```python
from build123d import *

# Parameters (mm, degrees)
SKETCH2_R           = 136
BOSS_EXTRUDE1_DEPTH = 8
SKETCH3_R           = 111.5
SKETCH3_R_2         = 108.5
CUT_EXTRUDE1_DEPTH  = 2
SKETCH4_R           = 3.3
CUT_EXTRUDE2_DEPTH  = 22
CIRPATTERN1_COUNT   = 6
SKETCH6_R           = 67.5
SKETCH6_R_2         = 55
BOSS_EXTRUDE2_DEPTH = 10
SKETCH7_R           = 3.3
CUT_EXTRUDE3_DEPTH  = 15
CIRPATTERN2_COUNT   = 6


with BuildPart() as part:
    # Sketch1 → Revolve1 (revolve)
    with BuildSketch(Plane.XY, mode=Mode.PRIVATE) as revolve1_sk:
        with BuildLine():
            Line((-65, 0), (-65, 5))
            Line((-65, 5), (-54.772255751, 5))
            ThreePointArc((-54.772255751, 5), (-37.080992435, 40.620192023), (0, 55))
            Line((0, 55), (0, 50))
            ThreePointArc((0, 50), (-35.355339059, 35.355339059), (-50, 0))
            Line((-50, 0), (-65, 0))
        make_face()
    revolve(revolve1_sk.sketch.rotate(Axis((0, 0, 0), (0, 1, 0)), 180), axis=Axis((0, 0, 0), (0, 1, 0)))

    # Sketch2 → Boss-Extrude1 (add)
    with BuildSketch(Plane(origin=(0, 0, 0), x_dir=(1, 0, 0), z_dir=(0, 1, 0))):
        with Locations(Location((0, 0, 0), (0, 0, 270))):
            Circle(SKETCH2_R)
    extrude(amount=BOSS_EXTRUDE1_DEPTH)

    # Sketch3 → Cut-Extrude1 (cut)
    with BuildSketch(Plane(origin=(0, 0, 0), x_dir=(1, 0, 0), z_dir=(0, 1, 0))):
        with Locations(Location((0, 0, 0), (0, 0, 180))):
            Circle(SKETCH3_R)
        with Locations(Location((0, 0, 0), (0, 0, 180))):
            Circle(SKETCH3_R_2, mode=Mode.SUBTRACT)
    extrude(amount=CUT_EXTRUDE1_DEPTH, mode=Mode.SUBTRACT)

    # Sketch4 → Cut-Extrude2 (cut)
    with BuildSketch(Plane(origin=(0, 0, 0), x_dir=(-1, 0, 0), z_dir=(0, -1, 0))):
        with Locations(Location((0, 121, 0), (0, 0, 180))):
            Circle(SKETCH4_R)
    cut_extrude2 = extrude(amount=-CUT_EXTRUDE2_DEPTH, mode=Mode.SUBTRACT)

    # CirPattern1: Cut-Extrude2 ×6 about axis
    cirpattern1_axis = Axis((0, 0, 0), (0, 1, 0))
    for i in range(1, CIRPATTERN1_COUNT):
        add(cut_extrude2.rotate(cirpattern1_axis, i * 360 / CIRPATTERN1_COUNT), mode=Mode.SUBTRACT)

    # Sketch6 → Boss-Extrude2 (add)
    with BuildSketch(Plane(origin=(0, 8, 0), x_dir=(1, 0, 0), z_dir=(0, 1, 0))):
        with Locations(Location((0, 0, 0), (0, 0, 270))):
            Circle(SKETCH6_R)
        with Locations(Location((0, 0, 0), (0, 0, 270))):
            Circle(SKETCH6_R_2, mode=Mode.SUBTRACT)
    extrude(amount=BOSS_EXTRUDE2_DEPTH)

    # Sketch7 → Cut-Extrude3 (cut)
    with BuildSketch(Plane(origin=(0, 18, 0), x_dir=(1, 0, 0), z_dir=(0, 1, 0))):
        with Locations(Location((0, -60, 0), (0, 0, 270))):
            Circle(SKETCH7_R)
    cut_extrude3 = extrude(amount=-CUT_EXTRUDE3_DEPTH, mode=Mode.SUBTRACT)

    # CirPattern2: Cut-Extrude3 ×6 about axis
    cirpattern2_axis = Axis((0, 0, 0), (0, 1, 0))
    for i in range(1, CIRPATTERN2_COUNT):
        add(cut_extrude3.rotate(cirpattern2_axis, i * 360 / CIRPATTERN2_COUNT), mode=Mode.SUBTRACT)


solid = part.part
```
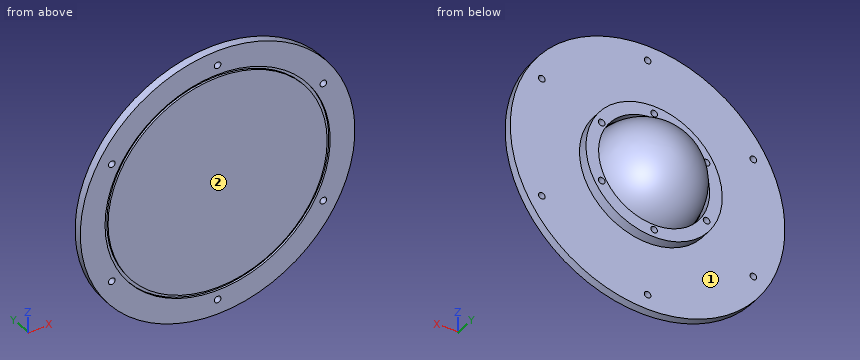
For this review, take the finished solid that the model builds, in its own axes (mm). Face numbers are marked on the shaded views. A direction names the side the tool comes from. Give positions to 0.01 mm unless a question says otherwise; leave off trailing zeros. Write each loop counter-clockwise with the first axis right and the second up, starting at its lowest first coordinate (ties: lowest second). Pieces come first, ordered by that corner, then holes.
Item 1: Take a section at B-B (z = 0). Give the boundary of the cut face in (x, y), and give its area (3 significant figures).
Item 2: Take a section at A-A (x = -34.5). Give the boundary of the cut face in (y, z).
Item 3: Take a section at D-D (z = -121). Give the boundary of the cut face in (x, y), and give its area (3 significant figures).
Item 4: Take a section at C-C (x = 0). Give the number of separate pieces and of enclosed holes in the cut face, and give its area (3 significant figures).
Item 5: Wall thickness on probe 1 along X at (y, z) = (10, 30); probe 2 along Y at (x, z) = (27.5, -63.5); probe 3 along Z at (x, y) = (-33, 13): over which ranges is each line inside the solid? List them lowest first.
Item 6: Machinability: for the marked faces 1 and 2, which of the approach directions +Z, -Z, +X, -X, +Y, -Y give a long, thin tool a straight path to every point of the face, cutting with its end or side? Answer none if there is none.
Item 7: Insertion check: P1, Ø7.5, axis at x = 0, z = -60, coming from the +Y side; P2, Ø8, axis at x = 70, z = 43.5, coming from the +Y side; P3, Ø4, axis at x = 51.96, z = -30, coming from the -Y side; P4, Ø2, axis at x = -52.5, z = 30, coming from the +Y side. Each pin has a flat end and moves straight along its axis. Give the tip position at first contact, or say it passes through.
Established:
1. outline: (-136, 0) - (-111.5, 0) - (-111.5, 2) - (-108.5, 2) - (-108.5, 0) - (108.5, 0) - (108.5, 2) - (111.5, 2) - (111.5, 0) - (136, 0) - (136, 8) - (67.5, 8) - (67.5, 18) - (55, 18) - (55, 8) - (54.42, 8) arc R55 ccw to (-54.42, 8) - (-55, 8) - (-55, 18) - (-67.5, 18) - (-67.5, 8) - (-136, 8) - close; hole (-49.36, 8) - (49.36, 8) arc R50 ccw to start
1. area: 3,160 mm2
2. outline: (0, -131.55) - (8, -131.55) - (8, -58.02) - (18, -58.02) - (18, -42.83) - (8, -42.83) - (8, -42.08) arc R42.83 ccw to (8, 42.08) - (8, 42.83) - (18, 42.83) - (18, 58.02) - (8, 58.02) - (8, 131.55) - (0, 131.55) - (0, 106.03) - (2, 106.03) - (2, 102.87) - (0, 102.87) - (0, -102.87) - (2, -102.87) - (2, -106.03) - (0, -106.03) - close; hole (8, -35.3) arc R36.19 ccw to (8, 35.3) - close
3. outline: (-62.09, 0) - (-3.3, 0) - (-3.3, 8) - (-62.09, 8) - close; (3.3, 0) - (62.09, 0) - (62.09, 8) - (3.3, 8) - close
3. area: 941 mm2
4. separate pieces: 3
4. enclosed holes: 1
4. area: 2,850 mm2
5. probe 1: x = -60.47 to -55.26, -48.66 to -46.1, -45 to -38.73, 38.73 to 45, 46.1 to 48.66, 55.26 to 60.47
5. probe 2: y = 0 to 8
5. probe 3: z = -58.88 to -44, -42.04 to -35.24, 35.24 to 42.04, 44 to 58.88
6. face 1: +Y
6. face 2: +Z, -Z, +X, -X, -Y
7. P1: stops at y = 18
7. P2: stops at y = 8
7. P3: stops at y = 0
7. P4: stops at y = 3
